Part model, mm, in its own coordinate system. A direction names the side the tool comes from. Round coordinates to 2 decimals unless told otherwise and drop trailing zeros. Loops run counter-clockwise (first coordinate to the right, second up) from the corner with the lowest first, then second, coordinate; pieces in that order, holes last. Notation, with made-up numbers: M -32,-10 L 1,-10 A32 ccw 1,20 Z; hole C -10,88 d5. An arc over 180 degrees is marked long. Answer as CSV lines item,"result". Start each with the question number.
Item 1: Band-saw the part on A-A (x = 0). Give the cut face in (y, z).
Item 2: Which spindle directions (+Z, -Z, +X, -X, +Y, -Y) get a long thin tool onto all of the face, cutting with end or side? Do faces 4 (the cylindrical face through (-0.759, -15.417, -0.951)), 5 (the cylindrical face through (-2.343, 17.847, 3.486)). Say none if no direction does.
Item 3: Mould opens along Y. For faces 1 (the cylindrical face through (-23.977, 1.055, -0.444)), 2 (the flat face through (5, 0, -4.5)), 3 (the cylindrical face through (-0.867, -3.905, -0.951)) say: pulls with the +Y half, pulls with the -Y half, needs draft (parallel to the pull), parting line crosses it, or undercut.
Item 4: Wall check: line 1 (Y direction, x = 0, z = -0.5); line 2 (Y direction, x = -2.5, z = -0.25); line 3 (Z direction, x = 7, y = 14.5). Give the ranges that are in metal, low to high.
Item 5: Drop flat-ended pins along their axis: pin 1 Ø1.5 at (x, z) = (2.5, -0.5) entering from +Y; pin 2 Ø4 at (x, y) = (-12, 0) entering from +Z (3 decimals); pin 3 Ø10 at (x, y) = (-6, 5) entering from +Z; pin 4 Ø4 at (y, z) = (16, 2.5) entering from +X. Give the stop position or say it passes through.
Item 6: Band-saw the part on B-B (z = -3.5). Give the cut face in (x, y), and give its area (3 significant figures).
```python
from build123d import *

# Parameters (mm, degrees)
SKETCH1_R           = 24
SKETCH1_R_2         = 18
BOSS_EXTRUDE3_DEPTH = 4.5
BOSS_EXTRUDE4_START = 2.5
SKETCH1_7_R         = 18
SKETCH1_7_R_2       = 16
SKETCH1_7_R_3       = 3.5
SKETCH1_7_R_4       = 4
BOSS_EXTRUDE4_DEPTH = 7
FILLET1_R           = 1


with BuildPart() as part:
    # Sketch1 → Boss-Extrude3 (new body, symmetric)
    with BuildSketch(Plane.XY):
        Circle(SKETCH1_R)
        Circle(SKETCH1_R_2, mode=Mode.SUBTRACT)
    extrude(amount=BOSS_EXTRUDE3_DEPTH, both=True)

    # Sketch1_7 → Boss-Extrude4 (add)
    with BuildSketch(Plane.XY.offset(BOSS_EXTRUDE4_START)):
        Circle(SKETCH1_7_R)
        Circle(SKETCH1_7_R_2, mode=Mode.SUBTRACT)
        Circle(SKETCH1_7_R_2)
        with Locations((12, 0)):
            Circle(SKETCH1_7_R_3, mode=Mode.SUBTRACT)
        with Locations((0, -12)):
            Circle(SKETCH1_7_R_3, mode=Mode.SUBTRACT)
        with Locations((-12, 0)):
            Circle(SKETCH1_7_R_3, mode=Mode.SUBTRACT)
        with Locations((0, 12)):
            Circle(SKETCH1_7_R_3, mode=Mode.SUBTRACT)
        Circle(SKETCH1_7_R_4, mode=Mode.SUBTRACT)
    extrude(amount=-BOSS_EXTRUDE4_DEPTH)

    # Fillet1
    fillet1_edges = [part.edges().sort_by_distance(p)[0] for p in [
        (-24, 0, 4.5),
    ]]
    fillet(fillet1_edges, radius=FILLET1_R)


solid = part.part
```
Answer block:
1,outline,"M -24,-4.5 L -15.5,-4.5 L -15.5,2.5 L -18,2.5 L -18,4.5 L -23,4.5 A1 ccw -24,3.5 Z; M -8.5,-4.5 L -4,-4.5 L -4,2.5 L -8.5,2.5 Z; M 4,-4.5 L 8.5,-4.5 L 8.5,2.5 L 4,2.5 Z; M 15.5,-4.5 L 24,-4.5 L 24,3.5 A1 ccw 23,4.5 L 18,4.5 L 18,2.5 L 15.5,2.5 Z"
2,face 4,"+Z, -Z"
2,face 5,"+Z"
3,face 1,"parting line crosses it"
3,face 2,"needs draft"
3,face 3,"undercut"
4,line 1,"y = -24 to -15.5, -8.5 to -4, 4 to 8.5, 15.5 to 24"
4,line 2,"y = -23.87 to -14.45, -9.55 to -3.12, 3.12 to 9.55, 14.45 to 23.87"
4,line 3,"z = -4.5 to 2.5"
5,pin 1,"stops at y = 23.94"
5,pin 2,"passes through"
5,pin 3,"stops at z = 2.5"
5,pin 4,"stops at x = 19.49"
6,outline,"C 0,0 d48; hole C -12,0 d7; hole C 0,0 d8; hole C 0,-12 d7; hole C 0,12 d7; hole C 12,0 d7"
6,area,"1,610 mm^2"
